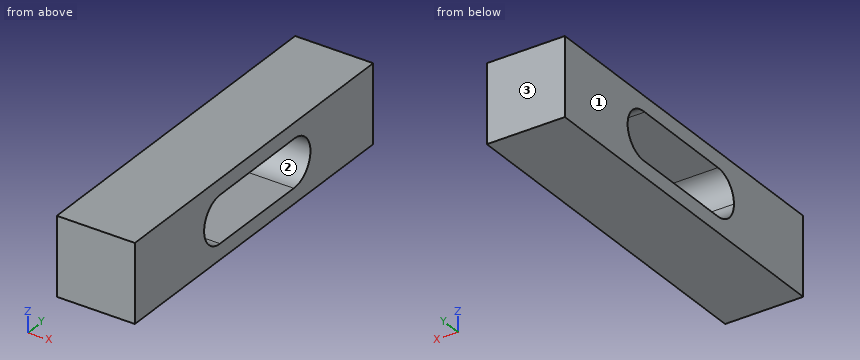
```python
from build123d import *

# Parameters (mm, degrees)
F0_W     = 12.717748
F0_H     = 12.717748
F1_DEPTH = 28.575
F3_DEPTH = 12.717748


with BuildPart() as f1:
    # F0 (on Front) → F1 (new body, symmetric)
    with BuildSketch(Plane.XZ):
        Rectangle(F0_W, F0_H)
    extrude(amount=F1_DEPTH, both=True)

    # F2 (on face) → F3 (cut, through all)
    with BuildSketch(Plane(origin=(-6.358874, 0, 0), x_dir=(0, -1, 0), z_dir=(-1, 0, 0))):
        with BuildLine():
            ThreePointArc((-9.433768, 3.872642), (-6.829732, 2.666259), (-5.767928, 0))
            ThreePointArc((-5.767928, 0), (-6.865206, -2.703241), (-9.536167, -3.876908))
            Line((-9.536167, -3.876908), (8.144981, -3.830927))
            ThreePointArc((8.144981, -3.830927), (4.304078, -0.000436), (8.144109, 3.830929))
            Line((8.144109, 3.830929), (-9.433768, 3.872642))
        make_face()
        with BuildLine():
            ThreePointArc((11.965958, 0), (10.847114, 2.705668), (8.144109, 3.830929))
            ThreePointArc((8.144109, 3.830929), (4.304078, -0.000436), (8.144981, -3.830927))
            ThreePointArc((8.144981, -3.830927), (10.847422, -2.705359), (11.965958, 0))
        make_face()
        with BuildLine():
            ThreePointArc((-9.536167, -3.876908), (-6.865206, -2.703241), (-5.767928, 0))
            ThreePointArc((-5.767928, 0), (-6.829732, 2.666259), (-9.433768, 3.872642))
            ThreePointArc((-9.433768, 3.872642), (-13.524539, 0.051244), (-9.536167, -3.876908))
        make_face()
    extrude(amount=-F3_DEPTH, mode=Mode.SUBTRACT)


solid = f1.part
```
For this review, take the finished solid that the model builds, in its own axes (mm). Face numbers are marked on the shaded views. Coordinates: 2 decimals unless noted, no trailing zeros. Loops run counter-clockwise (first coordinate to the right, second up) from the corner with the lowest first, then second, coordinate; pieces in that order, holes last.
1. For line 1 (Z direction, x = -1, y = -6.5); line 2 (Y direction, x = -1.5, z = 3) (3 decimals); line 3 (Y direction, x = 4.25, z = -3.5) (1 decimal), list the stretches that pass through material, from the lowest coordinate up.
2. Add section B-B, the plane y = 2.5. Give the boundary of the cut face in (x, z), then the cut area to 3 significant figures.
3. Add section C-C, the plane y = -7. Give the boundary of the cut face in (x, z), then the cut area to 3 significant figures.
4. Add section A-A, the plane x = -1. Give the boundary of the cut face in (y, z) (3 decimals), then the cut area to 3 significant figures.
5. Mouldability with a two-part tool opening along Y and no side actions: class the marked faces 1, 2 and 3 as +Y half, -Y half, draft (parallel to the pull), parting line (faces both ways), or undercut.
Result:
1. line 1: z = -6.36 to -3.84, 3.83 to 6.36
1. line 2: y = -28.575 to -10.517, 12.105 to 28.575
1. line 3: y = -28.6 to -9.7, 11.3 to 28.6
2. outline: (-6.36, -6.36) - (6.36, -6.36) - (6.36, -3.86) - (-6.36, -3.86) - close; (-6.36, 3.86) - (6.36, 3.86) - (6.36, 6.36) - (-6.36, 6.36) - close
2. area: 63.6 mm2
3. outline: (-6.36, -6.36) - (6.36, -6.36) - (6.36, -3.83) - (-6.36, -3.83) - close; (-6.36, 3.83) - (6.36, 3.83) - (6.36, 6.36) - (-6.36, 6.36) - close
3. area: 64.2 mm2
4. outline: (-28.575, -6.359) - (28.575, -6.359) - (28.575, 6.359) - (-28.575, 6.359) - close; hole (-11.966, 0) arc R3.831 ccw to (-8.145, -3.831) - (9.536, -3.877) arc R3.878 ccw (long way) to (9.434, 3.873) - (-8.144, 3.831) arc R3.831 ccw to start
4. area: 543 mm2
5. face 1: draft
5. face 2: undercut
5. face 3: +Y half
